Geometry: see drawing. Coordinates: mm, zero at the bounding-box minimum. Coordinates: 2 decimals unless noted, no trailing zeros. Loops run counter-clockwise (first coordinate to the right, second up) from the corner with the lowest first, then second, coordinate; pieces in that order, holes last. Notation, with made-up numbers: (57, -38) - (89, -38) arc R14 ccw to (89, -23) - close; hole circle Ø5 at (8, 33.5). An arc over 180 degrees is marked (long way). Use a Markdown table: item, result. Add a question column.
1. Section query A-A on z = 15. Return the cut outline in (x, y).
2. Ray query, L1, parallel to Z at x = 45, y = 1.9; L2, parallel to X at y = 0.9, z = 16.5. Return the intervals inside material, ascending. Write a range as [from, to].
3. Section query C-C on y = 1.5. State how many separate pieces and enclosed holes the cut face has, then the cut area to 3 significant figures.
4. Section query B-B on x = 35. Return the cut outline in (y, z), then the cut area to 3 significant figures.
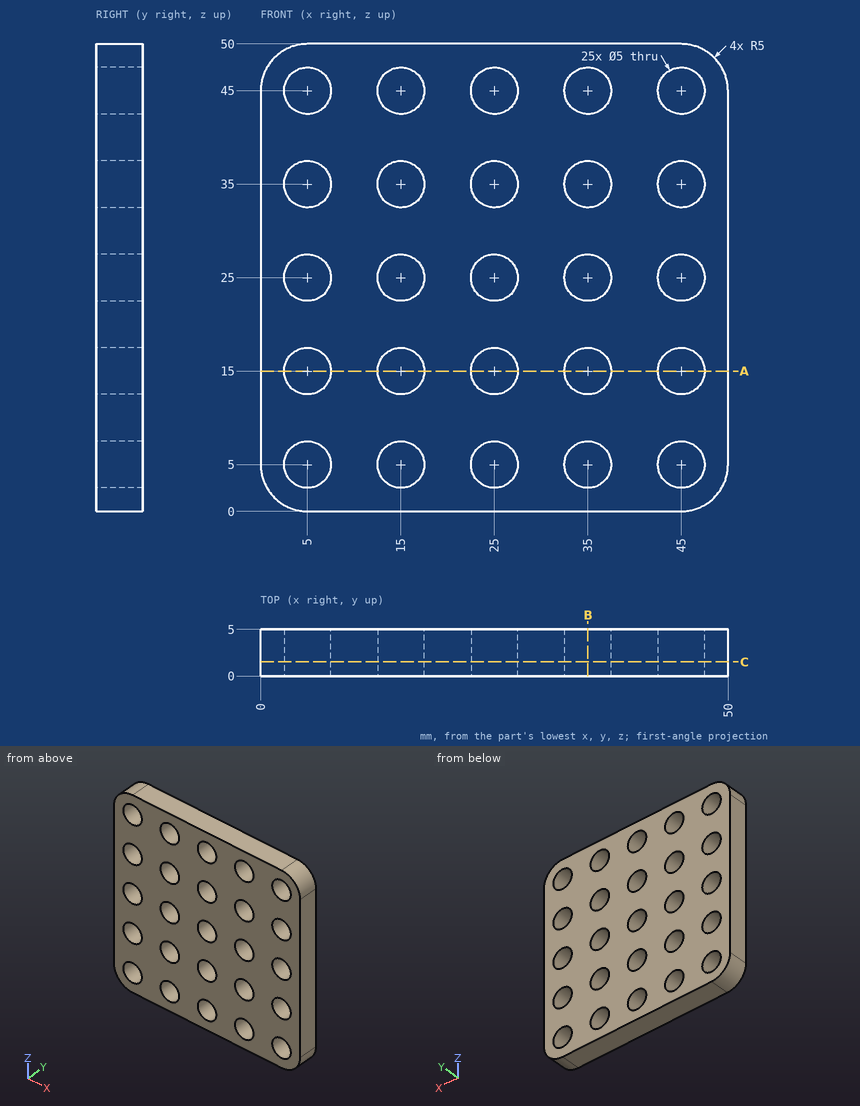
Resolved:
| question | item | result |
|---|---|---|
| 1 | outline | (0, 0) - (2.5, 0) - (2.5, 5) - (0, 5) - close; (7.5, 0) - (12.5, 0) - (12.5, 5) - (7.5, 5) - close; (17.5, 0) - (22.5, 0) - (22.5, 5) - (17.5, 5) - close; (27.5, 0) - (32.5, 0) - (32.5, 5) - (27.5, 5) - close; (37.5, 0) - (42.5, 0) - (42.5, 5) - (37.5, 5) - close; (47.5, 0) - (50, 0) - (50, 5) - (47.5, 5) - close |
| 2 | L1 | [0, 2.5], [7.5, 12.5], [17.5, 22.5], [27.5, 32.5], [37.5, 42.5], [47.5, 50] |
| 2 | L2 | [0, 3], [7, 13], [17, 23], [27, 33], [37, 43], [47, 50] |
| 3 | separate pieces | 1 |
| 3 | enclosed holes | 25 |
| 3 | area | 1,990 mm² |
| 4 | outline | (0, 0) - (5, 0) - (5, 2.5) - (0, 2.5) - close; (0, 7.5) - (5, 7.5) - (5, 12.5) - (0, 12.5) - close; (0, 17.5) - (5, 17.5) - (5, 22.5) - (0, 22.5) - close; (0, 27.5) - (5, 27.5) - (5, 32.5) - (0, 32.5) - close; (0, 37.5) - (5, 37.5) - (5, 42.5) - (0, 42.5) - close; (0, 47.5) - (5, 47.5) - (5, 50) - (0, 50) - close |
| 4 | area | 125 mm² |
